CAD build for the part. Positions are in the model's coordinates, mm. Face numbers are marked on the shaded views. A direction names the side the tool comes from. Give positions to 0.01 mm unless a question says otherwise; leave off trailing zeros. Loops run counter-clockwise (first coordinate to the right, second up) from the corner with the lowest first, then second, coordinate; pieces in that order, holes last. Notation, with made-up numbers: M 58.25,-1.75 L 97.25,-1.75 A10 cw 97.25,12.25 Z; hole C -40,29.5 d1. An arc over 180 degrees is marked long. Answer as CSV lines item,"result".
from build123d import *

# Parameters (mm, degrees)
F0_W     = 1219.2
F0_H     = 914.4
F1_DEPTH = 609.6
F2_T     = -25.4
F4_D     = 38.1
F6_D     = 38.1
F8_D     = 38.1


with BuildPart() as f1:
    # F0 (on Top) → F1 (new body)
    with BuildSketch(Plane.XY):
        with Locations((9.154483676, -105.9739306412)):
            Rectangle(F0_W, F0_H)
    extrude(amount=F1_DEPTH)

    # F2
    f2_openings = [f1.faces().sort_by_distance(p)[0] for p in [
        (9.154484, -105.973931, 609.6),
    ]]
    offset(amount=F2_T, openings=f2_openings)

    # F4 (through all)
    with Locations(Plane.XY.offset(25.4)):
        with Locations((-321.045516324, 109.9260693588), (339.354483676, 109.9260693588), (339.354483676, -321.8739306412), (-321.045516324, -321.8739306412), (0, -89.6527866654)):
            Hole(F4_D / 2)

    # F6 (through all)
    with Locations(Plane(origin=(0, 0, 0), x_dir=(1, 0, 0), z_dir=(0, 0, -1))):
        with Locations((0, -211.8932583313), (0, 423.8411196137)):
            Hole(F6_D / 2)

    # F8 (through all)
    with Locations(Plane(origin=(0, 0, 0), x_dir=(1, 0, 0), z_dir=(0, 0, -1))):
        with Locations((-473.445516324, 100.8939306412), (491.754483676, 100.8939306412)):
            Hole(F8_D / 2)


solid = f1.part
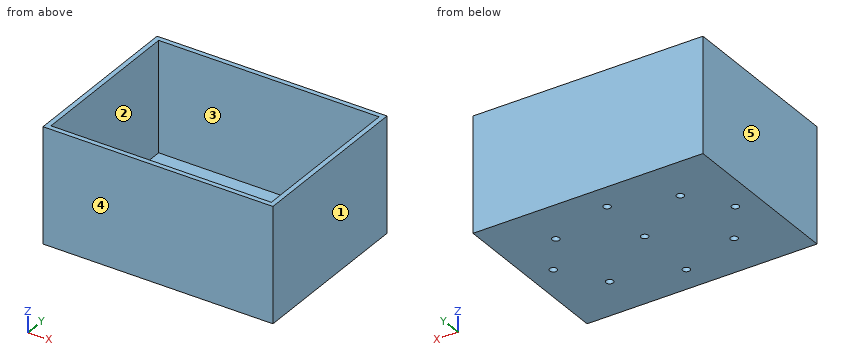
1) Band-saw the part on B-B on z = 298. Give the cut face in (x, y).
Answer below:
outline,"M -600.45,-563.17 L 618.75,-563.17 L 618.75,351.23 L -600.45,351.23 Z; hole M -575.05,-537.77 L 593.35,-537.77 L 593.35,325.83 L -575.05,325.83 Z"
2) Flat gauge pins, fed straight in: pin 1 (23 mm diameter, centred on x = 0, y = -423.84, fed in from -Z); pin 2 (6 mm diameter, centred on x = -455.5, y = 247, fed in from +Z). Where does each tip first touch, or does it go through?
Answer below:
pin 1,"passes through"
pin 2,"stops at z = 25.4"
3) Which spindle directions (+Z, -Z, +X, -X, +Y, -Y) get a long thin tool onto all of the face, cutting with end or side? Do the marked faces 1 and 2. Say none if no direction does.
Answer below:
face 1,"+Z, -Z, +X, +Y, -Y"
face 2,"+Z"
4) Band-saw the part on D-D on x = 215. Give the cut face in (y, z).
Answer below:
outline,"M -563.17,0 L 351.23,0 L 351.23,609.6 L 325.83,609.6 L 325.83,25.4 L -537.77,25.4 L -537.77,609.6 L -563.17,609.6 Z"
5) Drill centre lines: line 1 (Y direction, x = -116, z = 494.5); line 2 (X direction, y = 6, z = 124); line 3 (Y direction, x = 0, z = 8.5). Where is each one in solid material? Low to high. Write a range as from..to.
Answer below:
line 1,"y = -563.17..-537.77, 325.83..351.23"
line 2,"x = -600.45..-575.05, 593.35..618.75"
line 3,"y = -563.17..-442.89, -404.79..-108.7, -70.6..192.84, 230.94..351.23"
6) Mould opens along Y. For the marked faces 3, 4 and 5 say: +Y half, -Y half, draft (parallel to the pull), parting line (faces both ways), or undercut.
Answer below:
face 3,"undercut"
face 4,"-Y half"
face 5,"draft"
7) Band-saw the part on C-C on y = 152. Give the cut face in (x, z), and give its area (3 significant figures).
Answer below:
outline,"M -600.45,0 L 618.75,0 L 618.75,609.6 L 593.35,609.6 L 593.35,25.4 L -575.05,25.4 L -575.05,609.6 L -600.45,609.6 Z"
area,"60,600 mm^2"
8) Band-saw the part on A-A on x = 0. Give the cut face in (y, z).
Answer below:
outline,"M -563.17,0 L -442.89,0 L -442.89,25.4 L -537.77,25.4 L -537.77,609.6 L -563.17,609.6 Z; M -404.79,0 L -108.7,0 L -108.7,25.4 L -404.79,25.4 Z; M -70.6,0 L 192.84,0 L 192.84,25.4 L -70.6,25.4 Z; M 230.94,0 L 351.23,0 L 351.23,609.6 L 325.83,609.6 L 325.83,25.4 L 230.94,25.4 Z"
